Can you work these out from the model? Positions are in its coordinate system, mm. Round coordinates to 2 decimals unless told otherwise and drop trailing zeros. Loops run counter-clockwise (first coordinate to the right, second up) from the corner with the lowest first, then second, coordinate; pieces in that order, holes last. Notation, with made-up numbers: M 5.5,77 L 39.5,77 A19 cw 39.5,83 Z; hole C 5.5,80.5 d8. An arc over 180 degrees is marked long. Return JSON: item names as keys, results as strings.
```python
from build123d import *

# Parameters (mm, degrees)
SKETCH1_W               = 150
SKETCH1_H               = 150
BOSS_EXTRUDE1_DEPTH     = 1.5
CUT_EXTRUDE1_DEPTH      = 107.076623249
CUT_EXTRUDE1_DEPTH_BACK = 107.076623249
SKETCH2_R               = 2.75
CUT_EXTRUDE2_DEPTH      = 107.076623249
CUT_EXTRUDE2_DEPTH_BACK = 107.076623249
CUT_EXTRUDE3_DEPTH      = 107.076623249
CUT_EXTRUDE3_DEPTH_BACK = 107.076623249
SKETCH4_R               = 2.5
FILLET1_R               = 5


with BuildPart() as part:
    # Sketch1 → Boss-Extrude1 (new, symmetric)
    with BuildSketch(Plane.XY):
        Rectangle(SKETCH1_W, SKETCH1_H)
    extrude(amount=BOSS_EXTRUDE1_DEPTH, both=True)

    # Sketch2 → Cut-Extrude1 (cut, two sides: drawn at the far end of the back side and taken through both)
    with BuildSketch(Plane.XY.offset(-CUT_EXTRUDE1_DEPTH_BACK)):
        with Locations((0, 63.9)):
            Circle(SKETCH2_R)
        with Locations((63.9, 0)):
            Circle(SKETCH2_R)
        with Locations((0, -63.9)):
            Circle(SKETCH2_R)
        with Locations((-63.9, 0)):
            Circle(SKETCH2_R)
    extrude(amount=CUT_EXTRUDE1_DEPTH + CUT_EXTRUDE1_DEPTH_BACK, mode=Mode.SUBTRACT)

    # Sketch3 → Cut-Extrude2 (cut, two sides: drawn at the far end of the back side and taken through both)
    with BuildSketch(Plane.XY.offset(-CUT_EXTRUDE2_DEPTH_BACK)):
        with BuildLine():
            ThreePointArc((-56, -6.705221846), (0, -56.4), (56, -6.705221846))
            ThreePointArc((56, -6.705221846), (0, 56.4), (-56, -6.705221846))
        make_face()
    extrude(amount=CUT_EXTRUDE2_DEPTH + CUT_EXTRUDE2_DEPTH_BACK, mode=Mode.SUBTRACT)

    # Sketch4 → Cut-Extrude3 (cut, two sides: drawn at the far end of the back side and taken through both)
    with BuildSketch(Plane.XY.offset(-CUT_EXTRUDE3_DEPTH_BACK)):
        with Locations((-62.5, 50)):
            Circle(SKETCH4_R)
        with Locations(Location((-62.5, -50, 0), (0, 0, 180))):
            Circle(SKETCH4_R)
        with Locations((62.5, -50)):
            Circle(SKETCH4_R)
        with Locations(Location((62.5, 50, 0), (0, 0, 180))):
            Circle(SKETCH4_R)
    extrude(amount=CUT_EXTRUDE3_DEPTH + CUT_EXTRUDE3_DEPTH_BACK, mode=Mode.SUBTRACT)

    # Fillet1
    fillet1_edges = [part.edges().sort_by_distance(p)[0] for p in [
        (75, -75, 0),
        (-75, -75, 0),
        (-75, 75, 0),
        (75, 75, 0),
    ]]
    fillet(fillet1_edges, radius=FILLET1_R)


solid = part.part
```
Q1. If I drill on line 1 along X through (y, z) = (0, -0.6); line 2 along Y through (x, z) = (-62.5, -0.7), over which ranges is the centre line in solid material (lowest first)?
Results:
{"line 1": "x = -75 to -66.65, -61.15 to -56.4, 56.4 to 61.15, 66.65 to 75", "line 2": "y = -75 to -52.5, -47.5 to -2.37, 2.37 to 47.5, 52.5 to 75"}
Q2. Suppose I cut it at D-D, the plane y = 50. Please give me the cut outline in (x, z), plus the area to 3 significant figures.
Results:
{"outline": "M -75,-1.5 L -65,-1.5 L -65,1.5 L -75,1.5 Z; M -60,-1.5 L -26.1,-1.5 L -26.1,1.5 L -60,1.5 Z; M 26.1,-1.5 L 60,-1.5 L 60,1.5 L 26.1,1.5 Z; M 65,-1.5 L 75,-1.5 L 75,1.5 L 65,1.5 Z", "area": "263 mm2"}
Q3. Suppose I cut it at A-A, the plane z = 0.6. State how many separate pieces and enclosed holes the cut face has, plus the area to 3 significant figures.
Results:
{"separate pieces": "1", "enclosed holes": "9", "area": "12,300 mm2"}
Q4. Thinking about a two-plate mould opening in Y: for faces 1 (the cylindrical face through (-74, -73, 0)), 2 (the cylindrical face through (-61.28, 0.83, -0.02)), 3 (the flat face through (-34, 51, -1.5)), which applies, pulls with the +Y half, pulls with the -Y half, needs draft (parallel to the pull), parting line crosses it, or undercut?
Results:
{"face 1": "pulls with the -Y half", "face 2": "undercut", "face 3": "needs draft"}
Q5. Suppose I cut it at C-C, the plane x = 33. Please give me the cut outline in (y, z), plus the area to 3 significant figures.
Results:
{"outline": "M -75,-1.5 L -45.74,-1.5 L -45.74,1.5 L -75,1.5 Z; M 45.74,-1.5 L 75,-1.5 L 75,1.5 L 45.74,1.5 Z", "area": "176 mm2"}
Q6. I'm going to push flat-ended pins straight in: pin 1 Ø8 at (x, y) = (62.5, -50) entering from +Z; pin 2 Ø4.5 at (x, y) = (62.5, 50) entering from -Z. Where does each tip first touch, or does it pass through?
Results:
{"pin 1": "stops at z = 1.5", "pin 2": "passes through"}
Q7. Suppose I cut it at B-B, the plane y = -28.5. Please give me the cut outline in (x, z).
Results:
{"outline": "M -75,-1.5 L -48.67,-1.5 L -48.67,1.5 L -75,1.5 Z; M 48.67,-1.5 L 75,-1.5 L 75,1.5 L 48.67,1.5 Z"}
